The model under review builds one solid part; all positions refer to its coordinate system, in mm. A direction names the side the tool comes from. Round coordinates to 2 decimals unless told otherwise and drop trailing zeros. Order: outer loops, then holes, each group sorted by start corner. A loop starts at its lowest first (then second) coordinate and runs counter-clockwise, first axis right, second up. Notation, with made-up numbers: M -40,7 L 17,7 A21 ccw 17,27 Z; hole C -30.5,-17 d8. An arc over 180 degrees is marked long. Use a Markdown table: item, result. Add a question column.
1. Consider section D-D on y = 24. Count the separate pieces of the cut face and the enclosed holes in it, then the cut area to 3 significant figures.
2. Consider section B-B on z = 16.5. State the section outline as (x, y) points, then the cut area to 3 significant figures.
3. To check wall thickness, follow probe 1 along Y at (x, z) = (0, 37.75); probe 2 along X at (y, z) = (24, 39); probe 3 along Y at (x, z) = (0, 42). State the ranges of each line that lie inside material, in increasing order.
4. Consider section C-C on z = 37. State the section outline as (x, y) points.
5. Consider section A-A on y = 0. State the section outline as (x, z) points.
6. Insertion check: P1, Ø6, axis at y = 6, z = 21.5, coming from the -X side; P2, Ø1, axis at x = 8.5, y = -22, coming from the -Z side; P3, Ø1.5, axis at y = -21, z = 15, coming from the +X side; P4, Ø4, axis at x = 0, y = 24, coming from the +Z side. Each pin has a flat end and moves straight along its axis. Give the tip position at first contact, or say it passes through.
7. The part is to be moulded in two halves that separate along Y. For faces 1 (the flat face through (0, 0, 0)), 2 (the conical face through (-6.4, -28.81, 28.39)), 3 (the flat face through (3.4, 24, 39)), say which applies: +Y half, -Y half, draft (parallel to the pull), parting line (faces both ways), or undercut.
8. For faces 4 (the flat face through (-2, 25, 34.25)), 5 (the cylindrical face through (-0.487, 22.454, 39.18)), 6 (the flat face through (13, 25, 56)), list the 3-axis set-ups (+Z, -Z, +X, -X, +Y, -Y) from which the entire face can be reached by the end or side of a thin tool; tool diameter is ignored.
Solid Edge part; units mm, degrees
sketch "Sketch1" plane through (0, 0, 0) normal (0, -1, 0) x (1, 0, 0)
  line L0 (0, 0) -> (28.5, 0)
  line L1 (28.5, 0) -> (30.5, 56)
  line L2 (30.5, 56) -> (27.75, 56)
  line L3 (27.75, 56) -> (25.8482, 2.75)
  line L4 (25.8482, 2.75) -> (0, 2.75)
  line L5 (0, 2.75) -> (0, 0)
  dimension "D1" = 30.5
revolve "RevolvedProtrusion1" add sketch "Sketch1" angle 360 about axis through (0, 0, 54) along (0, 0, -1)
sketch "Sketch2" plane through (0, 0, 44.25) normal (0, 0, 1) x (1, 0, 0)
  line L0 (-3.4, 28.2965) -> (-3.4, 21.1)
  line L1 (-3.4, 21.1) -> (3.4, 21.1)
  line L2 (3.4, 21.1) -> (3.4, 28.2965)
  line L3 (-3.4, 28.2965) -> (3.4, 28.2965)
  dimension "D1" = 3.4
extrude "Ausprägung_1" add sketch "Sketch2" against normal blind 10
sketch "Sketch3" plane through (0, 0, 49.2) normal (0, 0, 1) x (1, 0, 0)
  line L0 (3.6, -28.2717) -> (3.6, -24.8)
  line L1 (-3.6, -28.2717) -> (-3.6, -24.8)
  arc A0 (3.6, -24.8) -> (-3.6, -24.8) centre (0, -24.8) ccw
  line L2 (3.6, -28.2717) -> (-3.6, -28.2717)
  dimension "D1" = 3.6
extrude "Ausprägung_2" add sketch "Sketch3" against normal up to next
hole "Bohrung_1" at (0, 24, 49.2) direction (0, 0, -1) diameter 3.242 depth 20 thread major 4 thread length 2
hole "Hole1" at (0, -24, 49.2) direction (0, 0, -1) diameter 3.242 depth 20 thread major 4 thread length 2
Answer block:
| question | item | result |
|---|---|---|
| 1 | separate pieces | 3 |
| 1 | enclosed holes | 0 |
| 1 | area | 690 mm^2 |
| 2 | outline | C 0,0 d58.18; hole M -3.6,-26.09 L -3.6,-24.8 A3.6 cw 3.6,-24.8 L 3.6,-26.09 A26.34 ccw long Z |
| 2 | area | 510 mm^2 |
| 3 | probe 1 | -29.85 to -25.62, -22.38 to -21.2, 21.1 to 22.38, 25.62 to 29.85 |
| 3 | probe 2 | -17.82 to -12.68, -3.4 to -1.62, 1.62 to 3.4, 12.68 to 17.82 |
| 3 | probe 3 | -30 to -25.62, -22.38 to -21.2, 21.1 to 22.38, 25.62 to 30 |
| 4 | outline | C 0,0 d59.64; hole M -3.6,-26.83 L -3.6,-24.8 A3.6 cw 3.6,-24.8 L 3.6,-26.83 A27.07 ccw 3.4,26.86 L 3.4,21.1 L -3.4,21.1 L -3.4,26.86 A27.07 ccw Z; hole C 0,-24 d3.24; hole C 0,24 d3.24 |
| 5 | outline | M -30.5,56 L -28.5,0 L 28.5,0 L 30.5,56 L 27.75,56 L 25.85,2.75 L -25.85,2.75 L -27.75,56 Z |
| 6 | P1 | x = -29.13 |
| 6 | P2 | z = 0 |
| 6 | P3 | x = 20.81 |
| 6 | P4 | z = 44.25 |
| 7 | face 1 | draft |
| 7 | face 2 | parting line |
| 7 | face 3 | undercut |
| 8 | face 4 | none |
| 8 | face 5 | +Z |
| 8 | face 6 | +Z, +X, -X, +Y, -Y |
